CAD build for the part. Positions are in the model's coordinates, mm. Face numbers are marked on the shaded views. A direction names the side the tool comes from. Round coordinates to 2 decimals unless told otherwise and drop trailing zeros. Order: outer loops, then holes, each group sorted by start corner. A loop starts at its lowest first (then second) coordinate and runs counter-clockwise, first axis right, second up. Notation, with made-up numbers: M 59,33 L 85,33 A17 cw 85,54 Z; hole C -11,-35 d11. An arc over 180 degrees is marked long. Answer as a JSON object with one key per item and string values.
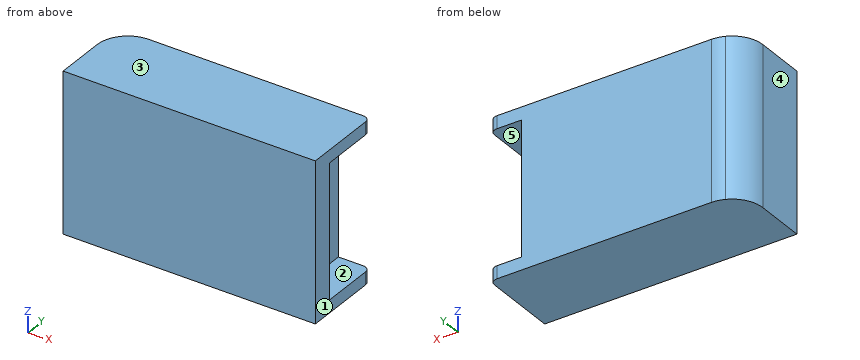
```python
from build123d import *

# Parameters (mm, degrees)
BOSS_EXTRUDE1_DEPTH = 31.75
SCREWHEADNOTCH_W    = 6.35
SCREWHEADNOTCH_H    = 26.67
CUT_EXTRUDE1_DEPTH  = 12


with BuildPart() as part:
    # Sketch1 → Boss-Extrude1 (new body)
    with BuildSketch(Plane.XY):
        with BuildLine():
            Line((-91.391382579, -26.616972455), (-141.791382579, -26.616972455))
            Line((-141.791382579, -26.616972455), (-141.791382579, -16.574195588))
            ThreePointArc((-141.791382579, -16.574195588), (-140.786841742, -13.20570186), (-138.101382579, -10.937627484))
            ThreePointArc((-138.101382579, -10.937627484), (-136.897886888, -10.553921764), (-135.641382579, -10.424195588))
            Line((-135.641382579, -10.424195588), (-92.778882579, -10.424195588))
            ThreePointArc((-92.778882579, -10.424195588), (-91.79777192, -10.83058493), (-91.391382579, -11.811695588))
            Line((-91.391382579, -11.811695588), (-91.391382579, -26.616972455))
        make_face()
    extrude(amount=-BOSS_EXTRUDE1_DEPTH)

    # ScrewHeadNotch → Cut-Extrude1 (cut)
    with BuildSketch(Plane(origin=(0, -10.424195588, 0), x_dir=(1, 0, 0), z_dir=(0, 1, 0))):
        with Locations((-94.566382579, 15.875)):
            Rectangle(SCREWHEADNOTCH_W, SCREWHEADNOTCH_H)
    extrude(amount=-CUT_EXTRUDE1_DEPTH, mode=Mode.SUBTRACT)


solid = part.part
```
Item 1: Drop flat-ended pins along their axis: pin 1 Ø6 at (x, y) = (-108, -17) entering from +Z; pin 2 Ø1 at (y, z) = (-13, -22.5) entering from +X; pin 3 Ø1.5 at (y, z) = (-15, -4) entering from -X; pin 4 Ø1.9 at (x, z) = (-93.5, -21.5) entering from +Y. Give the stop position or say it passes through.
Worked answers:
{"pin 1": "stops at z = 0", "pin 2": "stops at x = -97.74", "pin 3": "stops at x = -141.74", "pin 4": "stops at y = -22.42"}
Item 2: 3-axis set-ups, long thin cutter, end or side, ignore diameter. For the marked faces 4 and 5: which of +Z, -Z, +X, -X, +Y, -Y reach the whole face in a straight line?
Worked answers:
{"face 4": "+Z, -Z, -X, +Y, -Y", "face 5": "+X, +Y"}
Item 3: Saw through at B-B on z = -20. List the corners of the cut face in (x, y), and give its area (3 significant figures).
Worked answers:
{"outline": "M -141.79,-26.62 L -91.39,-26.62 L -91.39,-22.42 L -97.74,-22.42 L -97.74,-10.42 L -135.64,-10.42 A6.15 ccw -141.79,-16.57 Z", "area": "732 mm2"}
Item 4: Saw through at A-A on y = -20. List the corners of the cut face in (x, z), and give its area (3 significant figures).
Worked answers:
{"outline": "M -141.79,-31.75 L -91.39,-31.75 L -91.39,-29.21 L -97.74,-29.21 L -97.74,-2.54 L -91.39,-2.54 L -91.39,0 L -141.79,0 Z", "area": "1,430 mm2"}
Item 5: Two-plate mould, pull along Z, no slides. Class the marked faces 1, 2 and 3: released by +Z, released by -Z, zero draft, split by the parting line, or undercut.
Worked answers:
{"face 1": "zero draft", "face 2": "undercut", "face 3": "released by +Z"}
Item 6: Wall check: line 1 along X through (y, z) = (-18.25, -4); line 2 along X through (y, z) = (-13.5, -12). Give the ranges that are in metal, low to high. Write a range as [from, to].
Worked answers:
{"line 1": "x = [-141.79, -97.74]", "line 2": "x = [-140.97, -97.74]"}
